For this review, take the finished solid that the model builds, in its own axes (mm). Face numbers are marked on the shaded views. A direction names the side the tool comes from. Round coordinates to 2 decimals unless told otherwise and drop trailing zeros. Order: outer loops, then holes, each group sorted by start corner. A loop starts at its lowest first (then second) coordinate and runs counter-clockwise, first axis right, second up. Notation, with made-up numbers: M -26,41 L -21,41 A22 ccw -21,55 Z; hole C 71.5,-11 d2. An arc over 180 degrees is marked long. Put each result on its own line as item: value.
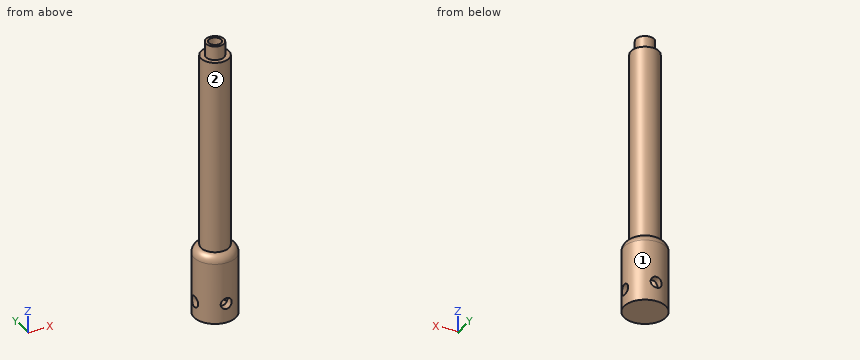
from build123d import *

# Parameters (mm, degrees)
F0_R      = 3.25
F0_R_2    = 2.25
F1_DEPTH  = 80
F0_R_3    = 5
F2_DEPTH  = 75
F0_R_4    = 7.5
F3_DEPTH  = 5
F4_DEPTH  = 20
F6_R      = 5.5
F7_DEPTH  = 2
F8_R      = 2
F9_DEPTH  = 12.5
F10_R     = 2
F11_DEPTH = 12.5


# Not quite as in the source:
# - a fillet or chamfer that OpenCascade refuses, or shapes differently, is made with other operations: its cross-section is extruded or revolved along the edge and cut away or added


with BuildPart() as f1:
    # F0 (on Top) → F1 (new body)
    with BuildSketch(Plane.XY):
        Circle(F0_R)
        Circle(F0_R_2, mode=Mode.SUBTRACT)
    extrude(amount=F1_DEPTH)

    # F0 (on Top) → F2 (join)
    with BuildSketch(Plane.XY):
        Circle(F0_R_3)
        Circle(F0_R, mode=Mode.SUBTRACT)
    extrude(amount=F2_DEPTH)

    # F0 (on Top) → F3 (join)
    with BuildSketch(Plane.XY):
        Circle(F0_R_4)
        Circle(F0_R_3, mode=Mode.SUBTRACT)
    extrude(amount=F3_DEPTH)

    # F0 (on Top) → F4 (join)
    with BuildSketch(Plane.XY):
        Circle(F0_R_4)
        Circle(F0_R_3, mode=Mode.SUBTRACT)
    extrude(amount=-F4_DEPTH)

    # F6 (on offset) → F7 (join)
    with BuildSketch(Plane(origin=(0, 0, -20), x_dir=(1, 0, 0), z_dir=(0, 0, -1))):
        Circle(F6_R)
    extrude(amount=-F7_DEPTH)

    # F8 (on Front) → F9 (cut, symmetric)
    with BuildSketch(Plane.XZ):
        with Locations((0, -13)):
            Circle(F8_R)
    extrude(amount=F9_DEPTH, both=True, mode=Mode.SUBTRACT)

    # F10 (on Right) → F11 (cut, symmetric)
    with BuildSketch(Plane.YZ):
        with Locations((0, -14)):
            Circle(F10_R)
    extrude(amount=F11_DEPTH, both=True, mode=Mode.SUBTRACT)

    # F12: fillet of radius 3 on 1 edges, made by hand

    # F12_s1 → F12_t2 (revolve, cut)
    with BuildSketch(Plane.XZ):
        with BuildLine():
            ThreePointArc((5, 5), (6.7912878475, 3.9784517816), (7.5, 2.0419601084))
            Line((7.5, 2.0419601084), (7.5, 5))
            Line((7.5, 5), (5, 5))
        make_face()
    revolve(axis=Axis((0, 0, 5), (0, 0, 1)), mode=Mode.SUBTRACT)


solid = f1.part
(1) Insertion check: pin 1 Ø2 at (y, z) = (3.5, 63) entering from +X; pin 2 Ø3 at (x, z) = (3.5, 55) entering from -Y; pin 3 Ø8 at (y, z) = (2, 52.5) entering from +X. Each pin has a flat end and moves straight along its axis. Give the tip position at first contact, or say it passes through.
A:
pin 1: stops at x = 4.33
pin 2: stops at y = -4.58
pin 3: stops at x = 5
(2) To check wall thickness, follow L1, parallel to X at y = 0, z = -5.25; L2, parallel to X at y = -0.25, z = 22. State the ranges of each line that lie inside material, in increasing order.
A:
L1: x = -7.5 to -5, 5 to 7.5
L2: x = -4.99 to -2.24, 2.24 to 4.99
(3) For the marked faces 1 and 2, list the 3-axis set-ups (+Z, -Z, +X, -X, +Y, -Y) from which the entire face can be reached by the end or side of a thin tool; tool diameter is ignored.
A:
face 1: +Z, -Z
face 2: +Z
(4) Add section C-C on z = 62.5. Give the boundary of the cut face in (x, y).
A:
outline: C 0,0 d10; hole C 0,0 d4.5
(5) Add section A-A on x = 0. Give the boundary of the cut face in (y, z).
A:
outline: M -7.5,-20 L 7.5,-20 L 7.5,-15 L 5,-15 L 5,-18 L -5,-18 L -5,-15 L -7.5,-15 Z; M -7.5,-11 L -5,-11 L -5,0 L -2.25,0 L -2.25,80 L -3.25,80 L -3.25,75 L -5,75 L -5,5 A3 ccw -7.5,2.04 Z; M 2.25,0 L 5,0 L 5,-11 L 7.5,-11 L 7.5,2.04 A3 ccw 5,5 L 5,75 L 3.25,75 L 3.25,80 L 2.25,80 Z
(6) Add section B-B on z = -13. Give the boundary of the cut face in (x, y), then the cut area to 3 significant figures.
A:
outline: M -7.3,-1.73 A7.5 ccw -2,-7.23 L -2,-4.58 A5 cw -4.69,-1.73 Z; M -7.3,1.73 L -4.69,1.73 A5 cw -2,4.58 L -2,7.23 A7.5 ccw Z; M 2,-7.23 A7.5 ccw 7.3,-1.73 L 4.69,-1.73 A5 cw 2,-4.58 Z; M 2,4.58 A5 cw 4.69,1.73 L 7.3,1.73 A7.5 ccw 2,7.23 Z
area: 60.2 mm2
